Can you work these out from the model? Positions are in its coordinate system, mm. A direction names the side the tool comes from. Give positions to 0.01 mm unless a question says otherwise; leave off trailing zeros. Loops run counter-clockwise (first coordinate to the right, second up) from the corner with the lowest first, then second, coordinate; pieces in that order, holes last.
from build123d import *

# Parameters (mm, degrees)
SKETCH1_W           = 16
SKETCH1_H           = 51
SKETCH1_R           = 3
BOSS_EXTRUDE1_DEPTH = 4
SKETCH2_R           = 8
BOSS_EXTRUDE2_DEPTH = 75
BOSS_EXTRUDE3_DEPTH = 2
SKETCH5_R           = 2.625
CUT_EXTRUDE1_DEPTH  = 35
FILLET1_R           = 5


with BuildPart() as part:
    # Sketch1 → Boss-Extrude1 (new body)
    with BuildSketch(Plane.XY):
        Rectangle(SKETCH1_W, SKETCH1_H)
        with Locations((0, 17.5)):
            Circle(SKETCH1_R, mode=Mode.SUBTRACT)
        with Locations((0, -17.5)):
            Circle(SKETCH1_R, mode=Mode.SUBTRACT)
    extrude(amount=BOSS_EXTRUDE1_DEPTH)

    # Sketch2 → Boss-Extrude2 (add)
    with BuildSketch(Plane.XY.offset(4)):
        Circle(SKETCH2_R)
    extrude(amount=BOSS_EXTRUDE2_DEPTH)

    # Sketch4 → Boss-Extrude3 (add)
    with BuildSketch(Plane(origin=(8, 0, 0), x_dir=(0, 0, -1), z_dir=(1, 0, 0))):
        Polygon((-4, 0), (-29.4, 0), (-4, -25.5), align=None)
    boss_extrude3 = extrude(amount=-BOSS_EXTRUDE3_DEPTH)

    # Mirror1: Boss-Extrude3 across plane
    add(boss_extrude3.mirror(Plane(origin=(0, 0, 0), x_dir=(0, 0, 1), z_dir=(1, 0, 0))))

    # Sketch5 → Cut-Extrude1 (cut)
    with BuildSketch(Plane.XY.offset(79)):
        Circle(SKETCH5_R)
    extrude(amount=-CUT_EXTRUDE1_DEPTH, mode=Mode.SUBTRACT)

    # Fillet1
    fillet1_edges = [part.edges().sort_by_distance(p)[0] for p in [
        (-8, 25.5, 2),
        (8, 25.5, 2),
    ]]
    fillet(fillet1_edges, radius=FILLET1_R)


solid = part.part
(1) Will these pins go through, and if not, where does the flat tip stop? P1, Ø1, axis at x = -1.5, z = 55, coming from the +Y side; P2, Ø6, axis at x = -6, z = 29.5, coming from the +Y side.
Returned:
P1: stops at y = 7.94
P2: stops at y = 7.42
(2) Suppose I cut it at C-C on z = 47.5. List the corners of the cut face in (x, y) for me (3 decimals).
Returned:
outline: circle Ø16 at (0, 0); hole circle Ø5.25 at (0, 0)
(3) Suppose I cut it at D-D on y = -19.5. List the corners of the cut face in (x, z) for me.
Returned:
outline: (-8, 0) - (-2.24, 0) - (-2.24, 4) - (-6, 4) - (-6, 9.98) - (-8, 9.98) - close; (2.24, 0) - (8, 0) - (8, 9.98) - (6, 9.98) - (6, 4) - (2.24, 4) - close
(4) Which directions (+Z, -Z, +X, -X, +Y, -Y) give clear straight access to the entire face, cutting with the end or side of a thin tool? Please do faces 5 (the cylindrical face through (-6.57, 24, 2.03)), 6 (the flat face through (-8, -7, 8)), 7 (the flat face through (6, -11, 10)), 8 (the cylindrical face through (-1.041, 7.932, 40.975)), 9 (the flat face through (-7.01, -15.4, 14.06)).
Returned:
face 5: +Z, -Z, -X, +Y
face 6: +Z, -Z, -X, +Y, -Y
face 7: +Z, -Y
face 8: +Z
face 9: +Z, -X, -Y
(5) Please list where these lines run through material, in increasing order: probe 1 along Y at (x, z) = (0, 2.3); probe 2 along Y at (x, z) = (0, 62) (3 decimals); probe 3 along Y at (x, z) = (0.5, 41.5).
Returned:
probe 1: y = -25.5 to -20.5, -14.5 to 14.5, 20.5 to 25.5
probe 2: y = -8 to -2.625, 2.625 to 8
probe 3: y = -7.98 to 7.98
(6) Thinking about a two-plate mould opening in Y: for faces 1 (the cylindrical face through (6.5, 24.07, 2.03)), 2 (the cylindrical face through (-0.65, 14.57, 1.97)), 3 (the flat face through (0, 0, 0)), 4 (the flat face through (7.01, -15.4, 14.06)), which applies, pulls with the +Y half, pulls with the -Y half, needs draft (parallel to the pull), parting line crosses it, or undercut?
Returned:
face 1: pulls with the +Y half
face 2: undercut
face 3: needs draft
face 4: pulls with the -Y half
(7) Suppose I cut it at A-A on x = 0. List the corners of the cut face in (y, z) for me (3 decimals).
Returned:
outline: (-25.5, 0) - (-20.5, 0) - (-20.5, 4) - (-25.5, 4) - close; (-14.5, 0) - (14.5, 0) - (14.5, 4) - (8, 4) - (8, 79) - (2.625, 79) - (2.625, 44) - (-2.625, 44) - (-2.625, 79) - (-8, 79) - (-8, 4) - (-14.5, 4) - close; (20.5, 0) - (25.5, 0) - (25.5, 4) - (20.5, 4) - close
(8) Suppose I cut it at B-B on y = 17.5. List the corners of the cut face in (x, z) for me.
Returned:
outline: (-8, 0) - (-3, 0) - (-3, 4) - (-8, 4) - close; (3, 0) - (8, 0) - (8, 4) - (3, 4) - close
